```python
from build123d import *

# Parameters (mm, degrees)
SKETCH1_R           = 2.5
BOSS_EXTRUDE1_DEPTH = 35
SKETCH2_R           = 2.5
SKETCH2_R_2         = 2
CUT_EXTRUDE1_DEPTH  = 8
SKETCH3_R           = 2.5
SKETCH3_R_2         = 2
CUT_EXTRUDE2_DEPTH  = 8
SKETCH4_R           = 2
BOSS_EXTRUDE2_DEPTH = 5


with BuildPart() as part:
    # Sketch1 → Boss-Extrude1 (new body, symmetric)
    with BuildSketch(Plane(origin=(0, 0, 0), x_dir=(0, 0, -1), z_dir=(1, 0, 0))):
        Circle(SKETCH1_R)
    extrude(amount=BOSS_EXTRUDE1_DEPTH, both=True)

    # Sketch2 → Cut-Extrude1 (cut)
    with BuildSketch(Plane(origin=(35, 0, 0), x_dir=(0, 0, -1), z_dir=(1, 0, 0))):
        Circle(SKETCH2_R)
        Circle(SKETCH2_R_2, mode=Mode.SUBTRACT)
    extrude(amount=-CUT_EXTRUDE1_DEPTH, mode=Mode.SUBTRACT)

    # Sketch3 → Cut-Extrude2 (cut)
    with BuildSketch(Plane.ZY.offset(35)):
        Circle(SKETCH3_R)
        Circle(SKETCH3_R_2, mode=Mode.SUBTRACT)
    extrude(amount=-CUT_EXTRUDE2_DEPTH, mode=Mode.SUBTRACT)

    # Sketch4 → Boss-Extrude2 (add)
    with BuildSketch(Plane(origin=(35, 0, 0), x_dir=(0, 0, -1), z_dir=(1, 0, 0))):
        Circle(SKETCH4_R)
    extrude(amount=BOSS_EXTRUDE2_DEPTH)


solid = part.part
```
Geometry check sheet. Reference: the model listing, model coordinates, mm. A direction names the side the tool comes from. Coordinates: 2 decimals unless noted, no trailing zeros. Write each loop counter-clockwise with the first axis right and the second up, starting at its lowest first coordinate (ties: lowest second). Pieces come first, ordered by that corner, then holes. Notation, with made-up numbers: M -1.75,52 L 20.25,52 A22 ccw 20.25,67 Z; hole C 6,72 d4. An arc over 180 degrees is marked long. Answer as a JSON object with one key per item and string values.
1. Section check A-A, the plane y = 0. Enter the section's corners in (x, z).
Answers below:
{"outline": "M -35,-2 L -27,-2 L -27,-2.5 L 27,-2.5 L 27,-2 L 40,-2 L 40,2 L 27,2 L 27,2.5 L -27,2.5 L -27,2 L -35,2 Z"}
2. Section check D-D, the plane x = 15. Enter the section's corners in (y, z), plus the area to 3 significant figures.
Answers below:
{"outline": "C 0,0 d5", "area": "19.6 mm²"}
3. Section check C-C, the plane x = 31.5. Enter the section's corners in (y, z), plus the area to 3 significant figures.
Answers below:
{"outline": "C 0,0 d4", "area": "12.6 mm²"}
4. Scan lines: L1, parallel to X at y = -2.2, z = -0.45; L2, parallel to Y at x = 22, z = 1.5; L3, parallel to Y at x = 17, z = 0.1. Record each from-to range of solid material in increasing order.
Answers below:
{"L1": "x = -27 to 27", "L2": "y = -2 to 2", "L3": "y = -2.5 to 2.5"}
5. Tool access check on faces 1 (the flat face through (-27, 2, -1)), 2 (the flat face through (-35, 0, 0)), 3 (the flat face through (27, 2, 1)). Record the directions out of +Z, -Z, +X, -X, +Y, -Y that give a thin tool (end or side, any length) a straight path to the whole face; none if there is none.
Answers below:
{"face 1": "-X", "face 2": "+Z, -Z, -X, +Y, -Y", "face 3": "+X"}
